Input: part model. Units: mm. Frame: model coordinates. A direction names the side the tool comes from. Coordinates: 2 decimals unless noted, no trailing zeros. Order: outer loops, then holes, each group sorted by start corner. A loop starts at its lowest first (then second) coordinate and runs counter-clockwise, first axis right, second up. Notation, with made-up numbers: (38.25, 12.25) -> (65.25, 12.25) arc R24 cw to (65.25, 43.25) -> close; hole circle Ø9 at (78, 64.25). An arc over 180 degrees is marked (long way). One line per item, written item: value. Start each with the question number.
from build123d import *

# Parameters (mm, degrees)
F0_W      = 2032
F0_H      = 1524
F1_DEPTH  = 381
F2_W      = 1397
F2_H      = 1524
F3_DEPTH  = 381
F4_W      = 762
F4_H      = 762
F5_DEPTH  = 127
F5_FACE_W = 762
F5_FACE_H = 762
F6_DEPTH  = 508


with BuildPart() as f1:
    # F0 (on Front) → F1 (new body)
    with BuildSketch(Plane.XZ):
        Rectangle(F0_W, F0_H)
    extrude(amount=F1_DEPTH)

    # F2 (on face) → F3 (join)
    with BuildSketch(Plane.XZ.offset(381)):
        with Locations((-317.5, 0)):
            Rectangle(F2_W, F2_H)
    extrude(amount=F3_DEPTH)

    # F4 (on face) → F5 (join)
    with BuildSketch(Plane.XZ.offset(762)):
        with Locations((-635, 381)):
            Rectangle(F4_W, F4_H)
    extrude(amount=F5_DEPTH)

    # F5_face (on face) → F6 (cut, through all)
    with BuildSketch(Plane(origin=(-635, -889, 381), x_dir=(1, 0, 0), z_dir=(0, -1, 0))):
        Rectangle(F5_FACE_W, F5_FACE_H)
    extrude(amount=-F6_DEPTH, mode=Mode.SUBTRACT)


solid = f1.part
1) Section query C-C, the plane y = -535. Return the cut outline in (x, z), plus the area to 3 significant figures.
2) Ray query, line 1 along Z through (x, y) = (-673, -655); line 2 along Y through (x, z) = (622, 463); line 3 along X through (y, z) = (-642.5, -228). Return the intervals inside material, ascending. Write a range as from..to.
3) Section query A-A, the plane z = 374. Return the cut outline in (x, y).
4) Access query for faces 1 (the flat face through (-640, -381, 386)), 2 (the flat face through (381, -569, -11)), 3 (the flat face through (-172, -762, -159)). Directions: +Z, -Z, +X, -X, +Y, -Y. A direction counts if a zero-diameter tool reaches every point of the face in a straight line with its end or side. Return the directions, or none.
5) Pin query (flat end, axial travel): pin 1 Ø5 at (y, z) = (-468.5, 8) entering from -X. Return the tip coordinate at first contact, or that it passes through.
6) Section query B-B, the plane x = -669. Return the cut outline in (y, z).
7) Section query D-D, the plane x = 408. Return the cut outline in (y, z).
Entries:
1. outline: (-1016, -762) -> (381, -762) -> (381, 762) -> (-254, 762) -> (-254, 0) -> (-1016, 0) -> close
1. area: 1,550,000 mm2
2. line 1: z = -762..0
2. line 2: y = -381..0
2. line 3: x = -1016..381
3. outline: (-1016, -381) -> (-254, -381) -> (-254, -762) -> (381, -762) -> (381, -381) -> (1016, -381) -> (1016, 0) -> (-1016, 0) -> close
4. face 1: +Z, -X, -Y
4. face 2: +Z, -Z, +X, -Y
4. face 3: +Z, -Z, +X, -X, -Y
5. pin 1: stops at x = -254
6. outline: (-762, -762) -> (0, -762) -> (0, 762) -> (-381, 762) -> (-381, 0) -> (-762, 0) -> close
7. outline: (-381, -762) -> (0, -762) -> (0, 762) -> (-381, 762) -> close
